The listing builds one solid part. Answer for the finished solid, in the listing's coordinates (mm). A direction names the side the tool comes from. Round coordinates to 2 decimals unless told otherwise and drop trailing zeros. Order: outer loops, then holes, each group sorted by start corner. A loop starts at its lowest first (then second) coordinate and runs counter-clockwise, first axis right, second up. Notation, with made-up numbers: M 64.25,57 L 77.25,57 A18 cw 77.25,81 Z; hole C -37.75,65.5 d7. An arc over 180 degrees is marked long. Put each result on its own line as item: value. Start each with the question number.
1. Each of these flat-tipped pins is pushed along its axis until it touches: pin 1 Ø0.6 at (y, z) = (-0.5, 42.5) entering from +X; pin 2 Ø0.6 at (y, z) = (-1, 42.5) entering from -X. Where does it stop, or does it pass through?
2. The part is cut by section C-C (x = -48.5). Give the vertices of the cut face in (y, z), then the cut area to 3 significant figures.
3. The mould has two halves that part along Z. Classify faces 1 (the face through (-41.399, -0.626, 35.233)), 2 (the face through (-45, 0, 41)), 3 (the face through (-30.65, -0.63, 24.77)), 4 (the face through (-33.61, -0.63, 49.87)): +Z half, -Z half, draft (parallel to the pull), parting line (faces both ways), or undercut.
4. The part is cut by section D-D (z = 46). Give the vertices of the cut face in (x, y).
5. Consider line 1 (X direction, y = -0.3, z = 27); line 2 (Z direction, x = -40.5, y = -0.4); line 3 (X direction, y = -0.6, z = 61). Determine where each line is inside the solid, lowest interval first.
6. The part is cut by section B-B (z = 27). Give the vertices of the cut face in (x, y), then the cut area to 3 significant figures.
7. The part is cut by section A-A (x = -34). Give the vertices of the cut face in (y, z).
8. Which of the six approach directions +Z, -Z, +X, -X, +Y, -Y give full straight-line access (tool end or side, diameter ignored) to faces 5 (the face through (-33.76, -0.63, 32.05)), 6 (the face through (-26.36, -0.63, 25.95))?
from build123d import *

# Parameters (mm, degrees)
F1_DEPTH = 1.27


# Not quite as in the source:
# - ends of sketch curves that miss each other by under 0.0002 mm in the source are joined


with BuildPart() as f1:
    # F0 (on Front) → F1 (new body)
    with BuildSketch(Plane.XZ):
        Polygon((-44.6418710053, 40.8897735178), (-44.6418710053, 33.3539977979), (-44.6297971524, 33.3609944811), (-43.2404409197, 34.166113231), (-39.5050764062, 36.3307215128), (-38.1157201735, 37.1358402628), (-38.1182953477, 38.7416174302), (-38.1217403313, 40.8897735313), (-38.1217487156, 40.8950016529), align=None)
        Polygon((-44.6539448582, 33.3609944811), (-44.6418710053, 33.3539977979), (-44.6418710053, 40.8897735178), (-51.161993295, 40.8950016529), (-51.161993295, 40.8897735178), (-51.1654466629, 38.7416174302), (-51.1680218371, 37.1358402628), (-49.7786656044, 36.3307215128), (-46.0433010909, 34.166113231), align=None)
        Polygon((-44.6418710053, 40.8897735178), (-38.1217487156, 40.8950016529), (-38.1217487156, 40.9002297812), (-38.1217487156, 43.0483886446), (-38.1217487156, 44.6541678769), (-39.5123943237, 45.4570574931), (-43.2512253972, 47.6156726199), (-44.6418710053, 48.418562236), align=None)
        Polygon((-51.161993295, 40.8950016529), (-44.6418710053, 40.8897735178), (-44.6418710053, 48.418562236), (-46.0325166134, 47.6156726199), (-49.7713476869, 45.4570574931), (-51.161993295, 44.6541678769), (-51.161993295, 43.0483886446), (-51.161993295, 40.9002297812), align=None)
        Polygon((-41.5661535928, 62.0498394063), (-44.6418710053, 63.8223188678), (-44.6418710053, 48.418562236), (-43.2512253972, 47.6156726199), align=None)
        Polygon((-44.6418710053, 48.418562236), (-44.6418710053, 63.8223188678), (-47.7175884178, 62.0498394063), (-46.0325166134, 47.6156726199), align=None)
        Polygon((-37.1105166727, 62.0498394063), (-44.6418710053, 66.3980688576), (-44.6418710053, 63.8223188678), (-41.5661535928, 62.0498394063), (-38.2213332575, 60.1222808724), align=None)
        Polygon((-44.6418710053, 63.8223188678), (-44.6418710053, 66.3980688576), (-52.1732253379, 62.0498394063), (-51.0624087531, 60.1222808724), (-47.7175884178, 62.0498394063), align=None)
        Polygon((-24.7788576939, 48.806157048), (-24.7757621839, 44.9456783996), (-22.5510392338, 44.9474622851), (-22.5510392338, 53.6439211877), (-30.1115337683, 58.0089747424), (-31.2206558067, 56.0879190201), (-27.8758354714, 54.1603604862), (-24.7817211845, 52.3772792439), align=None)
        Polygon((-38.1217487156, 43.0483886446), (-24.7788576939, 48.806157048), (-24.7817211845, 52.3772792439), (-27.8758354714, 54.1603604862), (-39.5123943237, 45.4570574931), (-38.1217487156, 44.6541678769), align=None)
        Polygon((-22.5445603606, 36.8675168429), (-24.7692833106, 36.8657329574), (-24.7661878006, 33.0052543089), (-24.76332431, 29.4341321131), (-27.8545751064, 27.6460911595), (-31.1962999317, 25.713171045), (-30.0840985392, 23.7938964823), (-22.5306139252, 28.1710691232), align=None)
        Polygon((-24.76332431, 29.4341321131), (-24.7661878006, 33.0052543089), (-38.1182953477, 38.7416174302), (-38.1157201735, 37.1358402628), (-39.5050764062, 36.3307215128), (-27.8545751064, 27.6460911595), align=None)
        Polygon((-44.6827784364, 15.3815109795), (-44.6418710053, 15.3578055115), (-44.6418710053, 33.3539977979), (-44.6539448582, 33.3609944811), (-46.0433010909, 34.166113231), (-47.7515186761, 19.7346673406), (-51.0932435014, 21.6675874551), (-52.2071498666, 19.7418128067), align=None)
        Polygon((-44.6418710053, 33.3539977979), (-44.6418710053, 15.3578055115), (-44.6009635742, 15.3815109795), (-37.076592144, 19.7418128067), (-38.1904985092, 21.6675874551), (-41.5322233345, 19.7346673406), (-43.2404409197, 34.166113231), (-44.6297971524, 33.3609944811), align=None)
        Polygon((-51.1654466629, 38.7416174302), (-64.5175542099, 33.0052543089), (-64.5204177006, 29.4341321131), (-61.4291669042, 27.6460911595), (-49.7786656044, 36.3307215128), (-51.1680218371, 37.1358402628), align=None)
        Polygon((-64.5144587, 36.8657329574), (-66.73918165, 36.8675168429), (-66.7531280854, 28.1710691232), (-59.1996434714, 23.7938964823), (-58.0874420789, 25.713171045), (-61.4291669042, 27.6460911595), (-64.5204177006, 29.4341321131), (-64.5175542099, 33.0052543089), align=None)
        Polygon((-64.5020208261, 52.3772792439), (-64.5048843167, 48.806157048), (-51.161993295, 43.0483886446), (-51.161993295, 44.6541678769), (-49.7713476869, 45.4570574931), (-61.4079065392, 54.1603604862), align=None)
        Polygon((-58.0630862039, 56.0879190201), (-59.1722082423, 58.0089747424), (-66.7327027768, 53.6439211877), (-66.7327027768, 44.9474622851), (-64.5079798267, 44.9456783996), (-64.5048843167, 48.806157048), (-64.5020208261, 52.3772792439), (-61.4079065392, 54.1603604862), align=None)
    extrude(amount=F1_DEPTH)


solid = f1.part
Resolved:
1. pin 1: x = -38.12
1. pin 2: x = -51.16
2. outline: M -1.27,17.59 L 0,17.59 L 0,20.17 L -1.27,20.17 Z; M -1.27,35.59 L 0,35.59 L 0,46.19 L -1.27,46.19 Z; M -1.27,61.6 L 0,61.6 L 0,64.17 L -1.27,64.17 Z
2. area: 20.0 mm2
3. face 1: undercut
3. face 2: draft
3. face 3: -Z half
3. face 4: undercut
4. outline: M -66.73,-1.27 L -64.51,-1.27 L -64.51,0 L -66.73,0 Z; M -58,-1.27 L -50.5,-1.27 L -50.5,0 L -58,0 Z; M -48.83,-1.27 L -40.45,-1.27 L -40.45,0 L -48.83,0 Z; M -38.79,-1.27 L -31.28,-1.27 L -31.28,0 L -38.79,0 Z; M -24.78,-1.27 L -22.55,-1.27 L -22.55,0 L -24.78,0 Z
5. line 1: -64.73 to -60.31, -46.89 to -42.39, -28.97 to -24.55
5. line 2: 17.76 to 20.33, 35.75 to 46.03, 61.44 to 64.01
5. line 3: -51.57 to -49.54, -47.6 to -41.69, -39.74 to -37.72
6. outline: M -64.73,-1.27 L -60.31,-1.27 L -60.31,0 L -64.73,0 Z; M -46.89,-1.27 L -42.39,-1.27 L -42.39,0 L -46.89,0 Z; M -28.97,-1.27 L -24.55,-1.27 L -24.55,0 L -28.97,0 Z
6. area: 16.9 mm2
7. outline: M -1.27,32.23 L 0,32.23 L 0,36.97 L -1.27,36.97 Z; M -1.27,44.83 L 0,44.83 L 0,49.58 L -1.27,49.58 Z
8. face 5: +Y, -Y
8. face 6: -Z, +X, +Y, -Y
